```python
from build123d import *

# Parameters (mm, degrees)
F0_W      = 444.5
F0_H      = 203.2
F1_DEPTH  = 12.7
F3_DEPTH  = 4.826
F4_W      = 6.35
F4_H      = 511.048
F5_DEPTH  = 68.2625
F7_DEPTH  = 19.05
F9_D      = 14.2875
F9_DEPTH  = 38.1
F10_W     = 114.3
F10_H     = 177.8
F10_R     = 4.826
F11_DEPTH = 12.7
F12_W     = 82.55
F12_H     = 101.6
F12_R     = 3.96875
F13_DEPTH = 50.8


with BuildPart() as f1:
    # F0 (on Top) → F1 (new body)
    with BuildSketch(Plane.XY):
        Rectangle(F0_W, F0_H)
    extrude(amount=-F1_DEPTH)

    # F2 (on Front) → F3 (join, symmetric)
    with BuildSketch(Plane.XZ):
        Polygon((203.2, -12.7), (-203.2, -12.7), (-203.2, -523.748), (25.4, -523.748), (203.2, -101.6), align=None)
    extrude(amount=F3_DEPTH, both=True)

    # F4 (on Front) → F5 (join, symmetric)
    with BuildSketch(Plane.XZ):
        with Locations((3.175, -268.224)):
            Rectangle(F4_W, F4_H)
    extrude(amount=F5_DEPTH, both=True)

    # F6 (on face) → F7 (join)
    with BuildSketch(Plane(origin=(0, 0, -523.748), x_dir=(1, 0, 0), z_dir=(0, 0, -1))):
        Polygon((25.4, 101.6), (-203.2, 101.6), (-203.2, 4.826), (-203.2, -4.826), (-203.2, -101.6), (25.4, -101.6), (25.4, -4.826), (25.4, 4.826), align=None)
    extrude(amount=F7_DEPTH)

    # F9
    with Locations(Plane(origin=(0, 0, -542.798), x_dir=(1, 0, 0), z_dir=(0, 0, -1))):
        with Locations((-95.25, 82.55), (-184.15, 82.55), (-95.25, -82.55), (-184.15, -82.55)):
            Hole(F9_D / 2, depth=F9_DEPTH)

    # F10 (on face) → F11 (join)
    with BuildSketch(Plane.XY):
        with Locations((-152.4, 0)):
            Rectangle(F10_W, F10_H)
        with Locations((-190.5, -61.976)):
            Circle(F10_R, mode=Mode.SUBTRACT)
        with Locations((-114.3, -61.976)):
            Circle(F10_R, mode=Mode.SUBTRACT)
        with Locations((-190.5, 61.976)):
            Circle(F10_R, mode=Mode.SUBTRACT)
        with Locations((-114.3, 61.976)):
            Circle(F10_R, mode=Mode.SUBTRACT)
    extrude(amount=F11_DEPTH)

    # F12 (on face) → F13 (join)
    with BuildSketch(Plane.XY):
        with Locations((172.339, 0)):
            Rectangle(F12_W, F12_H)
        with Locations((143.764, -31.75)):
            Circle(F12_R, mode=Mode.SUBTRACT)
        with Locations((178.816, -31.75)):
            Circle(F12_R, mode=Mode.SUBTRACT)
        with Locations((143.764, 31.75)):
            Circle(F12_R, mode=Mode.SUBTRACT)
        with Locations((178.816, 31.75)):
            Circle(F12_R, mode=Mode.SUBTRACT)
    extrude(amount=F13_DEPTH)


solid = f1.part
```
The listing builds one solid part. Answer for the finished solid, in the listing's coordinates (mm). A direction names the side the tool comes from. Give positions to 0.01 mm unless a question says otherwise; leave off trailing zeros. Write each loop counter-clockwise with the first axis right and the second up, starting at its lowest first coordinate (ties: lowest second). Pieces come first, ordered by that corner, then holes. Notation, with made-up numbers: (72, -38.75) - (130, -38.75) arc R30 cw to (130, -1.75) - close; hole circle Ø5 at (12.25, -18). An arc over 180 degrees is marked (long way). Use one line per item in the form item = value. Start each with the question number.
1) Flat-ended cylindrical pins translate along their axes: pin 1 Ø12.5 at (x, y) = (-114.3, -61.976) entering from +Z; pin 2 Ø3 at (x, y) = (-189.5, 61) entering from +Z; pin 3 Ø14 at (y, z) = (-5, 8) entering from -X. Find the tip coordinate at first contact, or state that the pin passes through.
2) Find section C-C on y = 13.5. Determine the outline of the cut face in (x, z), plus the area to 3 significant figures.
3) Find section B-B on z = -66.5. Determine the outline of the cut face in (x, y), plus the area to 3 significant figures.
4) A tool of negligible diameter and unlimited length cuts with its end or side. For faces 1 (the face through (131.064, -1, 25)), 2 (the face through (0, -37, -272)), 3 (the face through (-203.2, 0, -394)), 4 (the face through (-209.55, -1, 6)), from which of +Z, -Z, +X, -X, +Y, -Y can it reach the whole face along a straight path? Write none if from no direction.
5) Consider line 1 along Y through (x, z) = (-190.5, 3.75); line 2 along X through (y, z) = (-31, 30); line 3 along Z through (x, y) = (-100.5, 57.5). Determine where each line is inside the solid, lowest interval first. Write a range as from..to.
6) The mould has two halves that part along Y. Classify faces 5 (the face through (-153, -88.9, 6)), 6 (the face through (82, 4.826, -208)), 7 (the face through (-88.113, -82.864, -533.14)): pulls with the +Y half, pulls with the -Y half, needs draft (parallel to the pull), parting line crosses it, or undercut.
7) Find section D-D on x = 84.5. Determine the outline of the cut face in (y, z), plus the area to 3 significant figures.
8) Find section A-A on y = 82.55. Determine the outline of the cut face in (x, z), plus the area to 3 significant figures.
Geometry results:
q1.pin_1 = 12.7
q1.pin_2 = 0
q1.pin_3 = -209.55
q2.outline = (-222.25, -12.7) - (0, -12.7) - (0, -523.75) - (-203.2, -523.75) - (-203.2, -542.8) - (25.4, -542.8) - (25.4, -523.75) - (6.35, -523.75) - (6.35, -12.7) - (222.25, -12.7) - (222.25, 0) - (213.61, 0) - (213.61, 50.8) - (131.06, 50.8) - (131.06, 0) - (-95.25, 0) - (-95.25, 12.7) - (-209.55, 12.7) - (-209.55, 0) - (-222.25, 0) - close
q2.area = 18,900 mm2
q3.outline = (-203.2, -4.83) - (0, -4.83) - (0, -68.26) - (6.35, -68.26) - (6.35, -4.83) - (203.2, -4.83) - (203.2, 4.83) - (6.35, 4.83) - (6.35, 68.26) - (0, 68.26) - (0, 4.83) - (-203.2, 4.83) - close
q3.area = 4,730 mm2
q4.face_1 = +Z, +Y, -Y
q4.face_2 = -X, -Y
q4.face_3 = -Z, -X, +Y, -Y
q4.face_4 = +Z, -X, +Y, -Y
q5.line_1 = -88.9..-66.8, -57.15..57.15, 66.8..88.9
q5.line_2 = 131.06..139.87, 147.66..174.92, 182.71..213.61
q5.line_3 = -542.8..-523.75, -12.7..12.7
q6.face_5 = pulls with the -Y half
q6.face_6 = pulls with the +Y half
q6.face_7 = undercut
q7.outline = (-101.6, -12.7) - (-4.83, -12.7) - (-4.83, -383.43) - (4.83, -383.43) - (4.83, -12.7) - (101.6, -12.7) - (101.6, 0) - (-101.6, 0) - close
q7.area = 6,160 mm2
q8.outline = (-222.25, -12.7) - (222.25, -12.7) - (222.25, 0) - (-95.25, 0) - (-95.25, 12.7) - (-209.55, 12.7) - (-209.55, 0) - (-222.25, 0) - close; (-203.2, -542.8) - (-191.29, -542.8) - (-191.29, -523.75) - (-203.2, -523.75) - close; (-177.01, -542.8) - (-102.39, -542.8) - (-102.39, -523.75) - (-177.01, -523.75) - close; (-88.11, -542.8) - (25.4, -542.8) - (25.4, -523.75) - (-88.11, -523.75) - close
q8.area = 10,900 mm2
